Check sheet for the modelled part. Datum: model origin and axes. Units: mm. Face numbers are marked on the shaded views. Give positions to 0.01 mm unless a question says otherwise; leave off trailing zeros. Write each loop counter-clockwise with the first axis right and the second up, starting at its lowest first coordinate (ties: lowest second). Pieces come first, ordered by that corner, then holes. Notation, with made-up numbers: M 48.25,23 L 82.25,23 A24 cw 82.25,59 Z; hole C 62.25,-34 d7. An arc over 180 degrees is marked long. Write item = value, one per line. Start each with the question number.
1) Cross-section at A-A, the plane x = 1.5. Record the cut outline in (y, z), plus the area to 3 significant figures.
2) Scan lines: line 1 along Z through (x, y) = (-7.25, 0); line 2 along Y through (x, z) = (-8.25, 15); line 3 along Y through (x, z) = (1.5, 43.5). Record each from-to range of solid material in increasing order. Write a range as [from, to].
3) Mould release check, pull along Y, two halves, no side actions. Record for the marked faces 1, 2, 3 and 4: released by +Y, released by -Y, zero draft, split by the parting line, or undercut.
4) Cross-section at C-C, the plane z = 5. Record the cut outline in (x, y), plus the area to 3 significant figures.
5) Cross-section at D-D, the plane x = -7.75. Record the cut outline in (y, z).
6) Cross-section at B-B, the plane y = -2.5. Record the cut outline in (x, z).
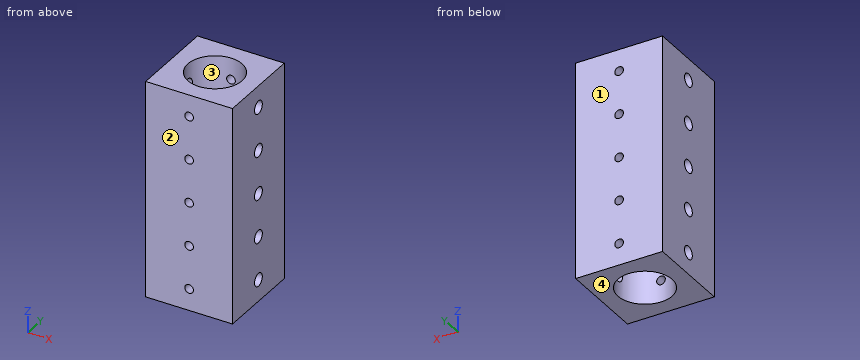
```python
from build123d import *

# Parameters (mm, degrees)
F0_W     = 20
F0_H     = 20
F0_R     = 6.25
F1_DEPTH = 50
F2_R     = 1.5
F3_DEPTH = 20
F4_R     = 1
F5_DEPTH = 20


with BuildPart() as f1:
    # F0 (on Top) → F1 (new body)
    with BuildSketch(Plane.XY):
        Rectangle(F0_W, F0_H)
        Circle(F0_R, mode=Mode.SUBTRACT)
    extrude(amount=F1_DEPTH)

    # F2 (on face) → F3 (cut, through all)
    with BuildSketch(Plane.YZ.offset(10)):
        with Locations((0, 45)):
            Circle(F2_R)
        with Locations((0, 35)):
            Circle(F2_R)
        with Locations((0, 25)):
            Circle(F2_R)
        with Locations((0, 15)):
            Circle(F2_R)
        with Locations((0, 5)):
            Circle(F2_R)
    extrude(amount=-F3_DEPTH, mode=Mode.SUBTRACT)

    # F4 (on face) → F5 (cut, through all)
    with BuildSketch(Plane.XZ.offset(10)):
        with Locations((0, 45)):
            Circle(F4_R)
        with Locations((0, 35)):
            Circle(F4_R)
        with Locations((0, 25)):
            Circle(F4_R)
        with Locations((0, 15)):
            Circle(F4_R)
        with Locations((0, 5)):
            Circle(F4_R)
    extrude(amount=-F5_DEPTH, mode=Mode.SUBTRACT)


solid = f1.part
```
Reply:
q1.outline = M -10,0 L -6.07,0 L -6.07,50 L -10,50 Z; M 6.07,0 L 10,0 L 10,50 L 6.07,50 Z
q1.area = 393 mm2
q2.line_1 = [0, 3.5], [6.5, 13.5], [16.5, 23.5], [26.5, 33.5], [36.5, 43.5], [46.5, 50]
q2.line_2 = [-10, -1.5], [1.5, 10]
q2.line_3 = [-10, -6.07], [6.07, 10]
q3.face_1 = released by +Y
q3.face_2 = released by -Y
q3.face_3 = undercut
q3.face_4 = zero draft
q4.outline = M -10,-10 L -1,-10 L -1,-6.17 A6.25 cw -6.07,-1.5 L -10,-1.5 Z; M -10,1.5 L -6.07,1.5 A6.25 cw -1,6.17 L -1,10 L -10,10 Z; M 1,-10 L 10,-10 L 10,-1.5 L 6.07,-1.5 A6.25 cw 1,-6.17 Z; M 1,6.17 A6.25 cw 6.07,1.5 L 10,1.5 L 10,10 L 1,10 Z
q4.area = 239 mm2
q5.outline = M -10,0 L 10,0 L 10,50 L -10,50 Z; hole C 0,5 d3; hole C 0,15 d3; hole C 0,25 d3; hole C 0,35 d3; hole C 0,45 d3
q6.outline = M -10,0 L -5.73,0 L -5.73,50 L -10,50 Z; M 5.73,0 L 10,0 L 10,50 L 5.73,50 Z
